```python
from build123d import *

# Parameters (mm, degrees)
SKETCH_1_W      = 43.5
SKETCH_1_H      = 18
EXTRUDE_1_DEPTH = 1.5
SKETCH_2_W      = 1.37636172
SKETCH_2_H      = 6.5
EXTRUDE_2_DEPTH = 3.8
SKETCH_3_W      = 9.5
SKETCH_3_H      = 7.5
EXTRUDE_7_DEPTH = 2.2
SKETCH_8_W      = 40.107603246
SKETCH_8_H      = 12.928280697
EXTRUDE_8_DEPTH = 2.5
SKETCH_9_W      = 14.27295549
SKETCH_9_H      = 7.021743376
EXTRUDE_9_DEPTH = 2.5


with BuildPart() as part:
    # Эскиз1 → Бобышка-Вытянуть1 (new body)
    with BuildSketch(Plane(origin=(0, 0, 0), x_dir=(1, 0, 0), z_dir=(0, 1, 0))):
        with Locations((21.75, 9)):
            Rectangle(SKETCH_1_W, SKETCH_1_H)
    extrude(amount=EXTRUDE_1_DEPTH)

    # Эскиз2 → Бобышка-Вытянуть2 (add)
    with BuildSketch(Plane(origin=(0, 1.5, 0), x_dir=(1, 0, 0), z_dir=(0, 1, 0))):
        with Locations((43.81181914, 9)):
            Rectangle(SKETCH_2_W, SKETCH_2_H)
    extrude(amount=EXTRUDE_2_DEPTH)

    # Эскиз3 → Бобышка-Вытянуть7 (add)
    with BuildSketch(Plane(origin=(0, 5.3, 0), x_dir=(1, 0, 0), z_dir=(0, 1, 0))):
        with Locations((39.75, 9)):
            Rectangle(SKETCH_3_W, SKETCH_3_H)
    extrude(amount=-EXTRUDE_7_DEPTH)

    # Эскиз8 → Бобышка-Вытянуть8 (add)
    with BuildSketch(Plane(origin=(0, 0, 0), x_dir=(-1, 0, 0), z_dir=(0, -1, 0))):
        with Locations((-22.53084927, 9.082336705)):
            Rectangle(SKETCH_8_W, SKETCH_8_H)
    extrude(amount=EXTRUDE_8_DEPTH)

    # Эскиз9 → Бобышка-Вытянуть9 (add)
    with BuildSketch(Plane(origin=(0, 1.5, 0), x_dir=(1, 0, 0), z_dir=(0, 1, 0))):
        with Locations((22.594203107, 8.908212505)):
            Rectangle(SKETCH_9_W, SKETCH_9_H)
    extrude(amount=EXTRUDE_9_DEPTH)


solid = part.part
```
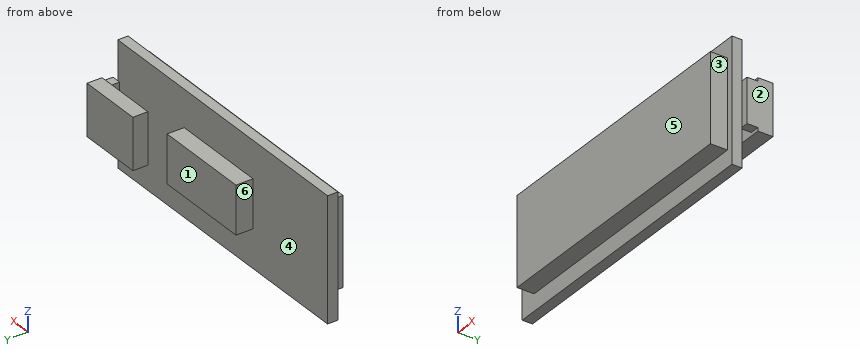
Geometry: final body of the model. Coordinates: model frame, mm. Face numbers are marked on the shaded views. A direction names the side the tool comes from. Coordinates: 2 decimals unless noted, no trailing zeros. Order: outer loops, then holes, each group sorted by start corner. A loop starts at its lowest first (then second) coordinate and runs counter-clockwise, first axis right, second up. Notation, with made-up numbers: M 76,48 L 108,48 A26 cw 108,73 Z; hole C 17,-22.75 d11. An arc over 180 degrees is marked long. Answer in a Markdown table with one row per item. Add a question column.
Q1. Reachability of the marked faces 1 and 2 from +Z, -Z, +X, -X, +Y, -Y: full face, straight path, thin tool, end or side. Return the list, or none.
Q2. Section query B-B on x = 40. Return the cut outline in (y, z).
Q3. Mould query, pull axis X, two halves, no side actions, for the marked faces 3, 4, 5 and 6. Classes: released by +X, released by -X, zero draft, split by the parting line, or undercut.
Q4. Section query C-C on x = 33.5. Return the cut outline in (y, z), and give its area (3 significant figures).
Q5. Contact query for flat-ended pins moving along their axis: P1, Ø0.5, axis at x = 44, z = -8, coming from the -Y side; P2, Ø9, axis at x = 29, z = -6.5, coming from the +Y side; P3, Ø2.5, axis at x = 42, y = 4.5, coming from the +Z side. Output: stop coordinate, or through.
Q6. Section query D-D on z = -14.75. Return the cut outline in (x, y), and give its area (3 significant figures).
Q7. Section query A-A on y = 3.5. Return the cut outline in (x, z).
Q8. Line query: L1, parallel to X at y = 2.75, z = -6; L2, parallel to Z at x = 40.5, y = -0.5; L3, parallel to Z at x = 28.5, y = 3.5. Output: solid intervals per line, ascending.
Completed:
| question | item | result |
|---|---|---|
| 1 | face 1 | +Z, -Z, -X, +Y |
| 1 | face 2 | +Z, -Z, +X, +Y, -Y |
| 2 | outline | M -2.5,-15.55 L 0,-15.55 L 0,-18 L 1.5,-18 L 1.5,0 L 0,0 L 0,-2.62 L -2.5,-2.62 Z; M 3.1,-12.75 L 5.3,-12.75 L 5.3,-5.25 L 3.1,-5.25 Z |
| 3 | face 3 | released by +X |
| 3 | face 4 | undercut |
| 3 | face 5 | zero draft |
| 3 | face 6 | released by -X |
| 4 | outline | M -2.5,-15.55 L 0,-15.55 L 0,-18 L 1.5,-18 L 1.5,0 L 0,0 L 0,-2.62 L -2.5,-2.62 Z |
| 4 | area | 59.3 mm2 |
| 5 | P1 | stops at y = 1.5 |
| 5 | P2 | stops at y = 4 |
| 5 | P3 | stops at z = -5.25 |
| 6 | outline | M 0,0 L 2.48,0 L 2.48,-2.5 L 42.58,-2.5 L 42.58,0 L 43.5,0 L 43.5,1.5 L 0,1.5 Z |
| 6 | area | 166 mm2 |
| 7 | outline | M 15.46,-12.42 L 29.73,-12.42 L 29.73,-5.4 L 15.46,-5.4 Z; M 35,-12.75 L 44.5,-12.75 L 44.5,-5.25 L 35,-5.25 Z |
| 8 | L1 | x = 15.46 to 29.73, 43.12 to 44.5 |
| 8 | L2 | z = -15.55 to -2.62 |
| 8 | L3 | z = -12.42 to -5.4 |
